CAD build for the part. Positions are in the model's coordinates, mm. A direction names the side the tool comes from. Coordinates: 2 decimals unless noted, no trailing zeros. Write each loop counter-clockwise with the first axis right and the second up, starting at its lowest first coordinate (ties: lowest second). Pieces come first, ordered by that corner, then holes. Notation, with made-up numbers: (56, -21) - (111, -21) arc R27 ccw to (111, 2) - close; hole circle Ø3 at (81, 87). An arc over 180 degrees is marked (long way). Answer in a Markdown table with one row per item. Add a question column.
Q1. Drill centre lines: line 1 along Y through (x, z) = (-39, 0); line 2 along Y through (x, z) = (-2, 0); line 3 along Z through (x, y) = (-29.5, 50.5). Where is each one in solid material? Low to high. Write a range as from..to.
Q2. Band-saw the part on C-C (z = 48). List the corners of the cut face in (x, y), and give its area (3 significant figures).
Q3. Band-saw the part on A-A (z = 0). List the corners of the cut face in (x, y).
Q4. Two-plate mould, pull along Z, no slides. Class faces 4 (the cylindrical face through (-2.96, 1.32, -29.97)), 5 (the flat face through (-22.093, -2.736, -31.267)), 6 (the flat face through (0, -24.3, 13.2)): +Z half, -Z half, draft (parallel to the pull), parting line (faces both ways), or undercut.
Q5. Pin check, flat tips, straight feed: pin 1 (1.5 mm diameter, centred on x = -34, y = 18, fed in from +Z); pin 2 (2 mm diameter, centred on x = -22, y = 39, fed in from -Z); pin 3 (4 mm diameter, centred on y = -6, z = -57.5, fed in from -X). Stop position of each tip, or through.
Q6. Band-saw the part on D-D (y = -15.5). State how many separate pieces and enclosed holes the cut face has, and give its area (3 significant figures).
Q7. Band-saw the part on B-B (x = -33). List the corners of the cut face in (y, z), and give its area (3 significant figures).
Q8. 3-axis set-ups, long thin cutter, end or side, ignore diameter. For faces 1 (the flat face through (-31, 44, 23)), 2 (the flat face through (-22.093, 28.446, 13.265)), 3 (the flat face through (-6, -22.3, 12.1)): which of +Z, -Z, +X, -X, +Y, -Y reach the whole face in a straight line?
```python
from build123d import *

# Parameters (mm, degrees)
SKETCH_5_R               = 30
SKETCH_5_R_2             = 27.5
EXTRUDE_1_DEPTH          = 6
REVOLVE_1_OUTLINE_W      = 67.5
REVOLVE_1_OUTLINE_H      = 2.5
REVOLVE_1_ANGLE          = 10
REVOLVE_2_ANGLE          = 5
PATTERN_CIRCULAR_1_COUNT = 3
EXTRUDE_2_DEPTH          = 10
EXTRUDE_2_DEPTH_BACK     = 20
SKETCH_14_R              = 81
SKETCH_14_R_2            = 75


# Read off the part's stored shape, not the designer's step: 旋轉1
with BuildPart() as part:
    # 草圖5 → 填料-伸長1 (new body)
    with BuildSketch(Plane.ZY):
        Circle(SKETCH_5_R)
        Circle(SKETCH_5_R_2, mode=Mode.SUBTRACT)
    extrude(amount=EXTRUDE_1_DEPTH)

    # 草圖13 → 旋轉3 (revolve)
    with BuildSketch(Plane(origin=(0, 0, 0), x_dir=(1, 0, 0), z_dir=(0, 1, 0))):
        Polygon((-6, 30), (-31, 7.5), (-25.444444444, 7.5), (-6, 25), align=None)
    revolve(axis=Axis((-1000, 0, 0), (1, 0, 0)))

    # 旋轉1 outline → 旋轉1 (revolve)
    with BuildSketch(Plane(origin=(0, 0, 0), x_dir=(0, -0.13052619222005293, -0.9914448613738103), z_dir=(0, -0.9914448613738103, 0.13052619222005293))):
        with Locations((41.25, -29.75)):
            Rectangle(REVOLVE_1_OUTLINE_W, REVOLVE_1_OUTLINE_H)
    revolve_1 = revolve(axis=Axis((0, 0, 0), (1, 0, 0)), revolution_arc=REVOLVE_1_ANGLE)

    # 草圖12 → 旋轉2 (revolve)
    with BuildSketch(Plane(origin=(0, 0, 0), x_dir=(1, 0, 0), z_dir=(0, 1, 0))):
        Polygon((-31, 54.917629386), (-6, 30), (-31, 7.5), align=None)
    revolve_2 = revolve(axis=Axis((0, 0, 0), (-1, 0, 0)), revolution_arc=REVOLVE_2_ANGLE)

    # 環狀複製排列1: 旋轉1, 旋轉2 ×3 about axis
    pattern_circular_1_axis = Axis((0, 0, 0), (1, 0, 0))
    add([revolve_1.rotate(pattern_circular_1_axis, i * 360 / PATTERN_CIRCULAR_1_COUNT) for i in range(1, PATTERN_CIRCULAR_1_COUNT)])
    add([revolve_2.rotate(pattern_circular_1_axis, i * 360 / PATTERN_CIRCULAR_1_COUNT) for i in range(1, PATTERN_CIRCULAR_1_COUNT)])

    # 草圖14 → 填料-伸長2 (add, two sides: drawn at the far end of the back side and taken through both)
    with BuildSketch(Plane(origin=(-28.5, 0, 0), x_dir=(0, 0, -1), z_dir=(1, 0, 0)).offset(-EXTRUDE_2_DEPTH_BACK)):
        Circle(SKETCH_14_R)
        Circle(SKETCH_14_R_2, mode=Mode.SUBTRACT)
    extrude(amount=EXTRUDE_2_DEPTH + EXTRUDE_2_DEPTH_BACK)


solid = part.part
```
Checked values:
| question | item | result |
|---|---|---|
| 1 | line 1 | y = -81..-75, 75..81 |
| 1 | line 2 | y = -30..-27.5, 27.5..30 |
| 1 | line 3 | z = -63.33..-55.45, 20.92..32.17, 55.45..63.33 |
| 2 | outline | (-48.5, -65.25) - (-18.5, -65.25) - (-18.5, -57.63) - (-48.5, -57.63) - close; (-48.5, 57.63) - (-18.5, 57.63) - (-18.5, 65.25) - (-48.5, 65.25) - close |
| 2 | area | 457 mm² |
| 3 | outline | (-48.5, -81) - (-18.5, -81) - (-18.5, -75) - (-48.5, -75) - close; (-48.5, 75) - (-18.5, 75) - (-18.5, 81) - (-48.5, 81) - close; (-31, -7.5) - (-6, -30) - (0, -30) - (0, -27.5) - (-6, -27.5) - (-6, -25) - (-25.44, -7.5) - close; (-31, 7.5) - (-25.44, 7.5) - (-6, 25) - (-6, 27.5) - (0, 27.5) - (0, 30) - (-6, 30) - close |
| 4 | face 4 | parting line |
| 4 | face 5 | undercut |
| 4 | face 6 | draft |
| 5 | pin 1 | stops at z = 79.14 |
| 5 | pin 2 | stops at z = -71.53 |
| 5 | pin 3 | stops at x = -31 |
| 6 | separate pieces | 3 |
| 6 | enclosed holes | 0 |
| 6 | area | 683 mm² |
| 7 | outline | circle Ø162 at (0, 0); hole circle Ø150 at (0, 0) |
| 7 | area | 2,940 mm² |
| 8 | face 1 | -X |
| 8 | face 2 | none |
| 8 | face 3 | +X |
